Input: part model. Units: mm. Frame: model coordinates. Face numbers are marked on the shaded views. A direction names the side the tool comes from. Round coordinates to 2 decimals unless told otherwise and drop trailing zeros. Order: outer loops, then holes, each group sorted by start corner. A loop starts at its lowest first (then second) coordinate and runs counter-clockwise, first axis right, second up. Notation, with made-up numbers: (-28.5, 73.5) - (5.5, 73.5) arc R21 cw to (5.5, 82.5) - close; hole circle Ø8 at (5, -28.75). An arc over 180 degrees is marked (long way). One line per item, written item: value. Start each with the question number.
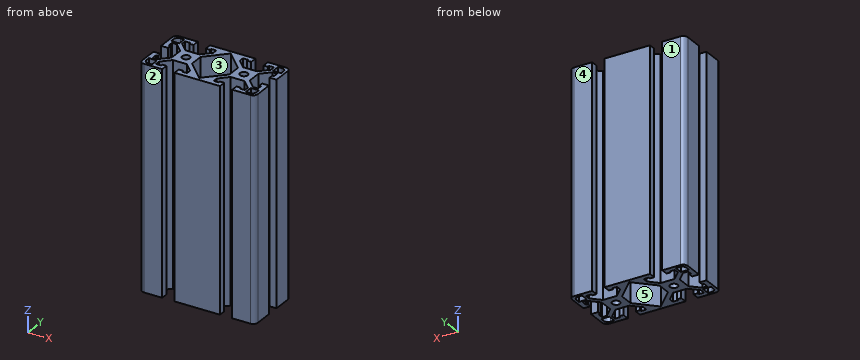
from build123d import *

# Parameters (mm, degrees)
SKETCH1_R           = 2.5527
BOSS_EXTRUDE1_DEPTH = 73.025


with BuildPart() as part:
    # Sketch1 → Boss-Extrude1 (new, symmetric)
    with BuildSketch(Plane.XY):
        with BuildLine():
            Line((-29.337, 12.442261469), (-29.337, 15.6718))
            Line((-29.337, 15.6718), (-25.908, 15.6718))
            Line((-25.908, 15.6718), (-25.908, 14.5034))
            Line((-25.908, 14.5034), (-23.114, 14.5034))
            Line((-23.114, 14.5034), (-23.114, 19.05))
            Line((-23.114, 19.05), (-35.052, 19.05))
            ThreePointArc((-35.052, 19.05), (-37.207261469, 18.157261469), (-38.1, 16.002))
            Line((-38.1, 16.002), (-38.1, 4.064))
            Line((-38.1, 4.064), (-33.5534, 4.064))
            Line((-33.5534, 4.064), (-33.5534, 6.858))
            Line((-33.5534, 6.858), (-34.7218, 6.858))
            Line((-34.7218, 6.858), (-34.7218, 10.287))
            Line((-34.7218, 10.287), (-31.492261469, 10.287))
            Line((-31.492261469, 10.287), (-25.781, 4.575738531))
            Line((-25.781, 4.575738531), (-25.781, -4.575738531))
            Line((-25.781, -4.575738531), (-31.492261469, -10.287))
            Line((-31.492261469, -10.287), (-34.7218, -10.287))
            Line((-34.7218, -10.287), (-34.7218, -6.858))
            Line((-34.7218, -6.858), (-33.5534, -6.858))
            Line((-33.5534, -6.858), (-33.5534, -4.064))
            Line((-33.5534, -4.064), (-38.1, -4.064))
            Line((-38.1, -4.064), (-38.1, -16.002))
            ThreePointArc((-38.1, -16.002), (-37.207261469, -18.157261469), (-35.052, -19.05))
            Line((-35.052, -19.05), (-23.114, -19.05))
            Line((-23.114, -19.05), (-23.114, -14.5034))
            Line((-23.114, -14.5034), (-25.908, -14.5034))
            Line((-25.908, -14.5034), (-25.908, -15.6718))
            Line((-25.908, -15.6718), (-29.337, -15.6718))
            Line((-29.337, -15.6718), (-29.337, -12.442261469))
            Line((-29.337, -12.442261469), (-23.625738531, -6.731))
            Line((-23.625738531, -6.731), (-14.474261469, -6.731))
            Line((-14.474261469, -6.731), (-8.763, -12.442261469))
            Line((-8.763, -12.442261469), (-8.763, -15.6718))
            Line((-8.763, -15.6718), (-12.192, -15.6718))
            Line((-12.192, -15.6718), (-12.192, -14.5034))
            Line((-12.192, -14.5034), (-14.986, -14.5034))
            Line((-14.986, -14.5034), (-14.986, -19.05))
            Line((-14.986, -19.05), (14.986, -19.05))
            Line((14.986, -19.05), (14.986, -14.5034))
            Line((14.986, -14.5034), (12.192, -14.5034))
            Line((12.192, -14.5034), (12.192, -15.6718))
            Line((12.192, -15.6718), (8.763, -15.6718))
            Line((8.763, -15.6718), (8.763, -12.442261469))
            Line((8.763, -12.442261469), (14.474261469, -6.731))
            Line((14.474261469, -6.731), (23.625738531, -6.731))
            Line((23.625738531, -6.731), (29.337, -12.442261469))
            Line((29.337, -12.442261469), (29.337, -15.6718))
            Line((29.337, -15.6718), (25.908, -15.6718))
            Line((25.908, -15.6718), (25.908, -14.5034))
            Line((25.908, -14.5034), (23.114, -14.5034))
            Line((23.114, -14.5034), (23.114, -19.05))
            Line((23.114, -19.05), (35.052, -19.05))
            ThreePointArc((35.052, -19.05), (37.207261469, -18.157261469), (38.1, -16.002))
            Line((38.1, -16.002), (38.1, -4.064))
            Line((38.1, -4.064), (33.5534, -4.064))
            Line((33.5534, -4.064), (33.5534, -6.858))
            Line((33.5534, -6.858), (34.7218, -6.858))
            Line((34.7218, -6.858), (34.7218, -10.287))
            Line((34.7218, -10.287), (31.492261469, -10.287))
            Line((31.492261469, -10.287), (25.781, -4.575738531))
            Line((25.781, -4.575738531), (25.781, 4.575738531))
            Line((25.781, 4.575738531), (31.492261469, 10.287))
            Line((31.492261469, 10.287), (34.7218, 10.287))
            Line((34.7218, 10.287), (34.7218, 6.858))
            Line((34.7218, 6.858), (33.5534, 6.858))
            Line((33.5534, 6.858), (33.5534, 4.064))
            Line((33.5534, 4.064), (38.1, 4.064))
            Line((38.1, 4.064), (38.1, 16.002))
            ThreePointArc((38.1, 16.002), (37.207261469, 18.157261469), (35.052, 19.05))
            Line((35.052, 19.05), (23.114, 19.05))
            Line((23.114, 19.05), (23.114, 14.5034))
            Line((23.114, 14.5034), (25.908, 14.5034))
            Line((25.908, 14.5034), (25.908, 15.6718))
            Line((25.908, 15.6718), (29.337, 15.6718))
            Line((29.337, 15.6718), (29.337, 12.442261469))
            Line((29.337, 12.442261469), (23.625738531, 6.731))
            Line((23.625738531, 6.731), (14.474261469, 6.731))
            Line((14.474261469, 6.731), (8.763, 12.442261469))
            Line((8.763, 12.442261469), (8.763, 15.6718))
            Line((8.763, 15.6718), (12.192, 15.6718))
            Line((12.192, 15.6718), (12.192, 14.5034))
            Line((12.192, 14.5034), (14.986, 14.5034))
            Line((14.986, 14.5034), (14.986, 19.05))
            Line((14.986, 19.05), (-14.986, 19.05))
            Line((-14.986, 19.05), (-14.986, 14.5034))
            Line((-14.986, 14.5034), (-12.192, 14.5034))
            Line((-12.192, 14.5034), (-12.192, 15.6718))
            Line((-12.192, 15.6718), (-8.763, 15.6718))
            Line((-8.763, 15.6718), (-8.763, 12.442261469))
            Line((-8.763, 12.442261469), (-14.474261469, 6.731))
            Line((-14.474261469, 6.731), (-23.625738531, 6.731))
            Line((-23.625738531, 6.731), (-29.337, 12.442261469))
        make_face()
        with Locations((-19.05, 0)):
            Circle(SKETCH1_R, mode=Mode.SUBTRACT)
        with Locations((19.05, 0)):
            Circle(SKETCH1_R, mode=Mode.SUBTRACT)
        Polygon((-12.319, 4.575738531), (-12.319, -4.575738531), (0, -16.894738531), (12.319, -4.575738531), (12.319, 4.575738531), (0, 16.894738531), align=None, mode=Mode.SUBTRACT)
        with BuildLine():
            Line((-30.9372, 11.8872), (-30.9372, 17.272))
            Line((-30.9372, 17.272), (-33.528, 17.272))
            ThreePointArc((-33.528, 17.272), (-35.503656347, 16.453656347), (-36.322, 14.478))
            Line((-36.322, 14.478), (-36.322, 11.8872))
            Line((-36.322, 11.8872), (-30.9372, 11.8872))
        make_face(mode=Mode.SUBTRACT)
        with BuildLine():
            Line((-30.9372, -17.272), (-30.9372, -11.8872))
            Line((-30.9372, -11.8872), (-36.322, -11.8872))
            Line((-36.322, -11.8872), (-36.322, -14.478))
            ThreePointArc((-36.322, -14.478), (-35.503656347, -16.453656347), (-33.528, -17.272))
            Line((-33.528, -17.272), (-30.9372, -17.272))
        make_face(mode=Mode.SUBTRACT)
        with BuildLine():
            Line((36.322, -11.8872), (30.9372, -11.8872))
            Line((30.9372, -11.8872), (30.9372, -17.272))
            Line((30.9372, -17.272), (33.528, -17.272))
            ThreePointArc((33.528, -17.272), (35.503656347, -16.453656347), (36.322, -14.478))
            Line((36.322, -14.478), (36.322, -11.8872))
        make_face(mode=Mode.SUBTRACT)
        with BuildLine():
            Line((30.9372, 17.272), (30.9372, 11.8872))
            Line((30.9372, 11.8872), (36.322, 11.8872))
            Line((36.322, 11.8872), (36.322, 14.478))
            ThreePointArc((36.322, 14.478), (35.503656347, 16.453656347), (33.528, 17.272))
            Line((33.528, 17.272), (30.9372, 17.272))
        make_face(mode=Mode.SUBTRACT)
    extrude(amount=BOSS_EXTRUDE1_DEPTH, both=True)


solid = part.part
Item 1: First-contact query: pin 1 Ø3.5 at (y, z) = (18, -25.5) entering from -X; pin 2 Ø4.5 at (x, z) = (-20.5, 10) entering from -Y; pin 3 Ø2.5 at (y, z) = (-2.5, 8) entering from -X. Flat tips, straight axial feed; report the tip coordinate or a pass-through.
Item 2: Section query B-B on y = 0. Return loops of the section in (x, z) (3 decimals).
Item 3: Section query C-C on z = -32.5. Give the number of separate pieces and of enclosed holes in the cut face, and give its area (3 significant figures).
Item 4: Line query: L1, parallel to Y at x = 33, z = 40; L2, parallel to Y at x = 14.5, z = 4.5; L3, parallel to Y at x = -19, z = 13. Output: solid intervals per line, ascending.
Item 5: Pull-direction query (Y, two-part tool) for the marked faces 1, 2 and 3; classes: released by +Y, released by -Y, zero draft, split by the parting line, or undercut.
Item 6: Section query D-D on x = -4. Return loops of the section in (y, z) (3 decimals), and give its area (3 significant figures).
Item 7: Section query A-A on x = 19.05. Return loops of the section in (y, z) (3 decimals).
Item 8: Reachability of the marked faces 4 and 5 from +Z, -Z, +X, -X, +Y, -Y: full face, straight path, thin tool, end or side. Return the list, or none.
Geometry results:
1. pin 1: stops at x = -38.09
1. pin 2: stops at y = -6.73
1. pin 3: stops at x = -25.78
2. outline: (-25.781, -73.025) - (-21.603, -73.025) - (-21.603, 73.025) - (-25.781, 73.025) - close; (-16.497, -73.025) - (-12.319, -73.025) - (-12.319, 73.025) - (-16.497, 73.025) - close; (12.319, -73.025) - (16.497, -73.025) - (16.497, 73.025) - (12.319, 73.025) - close; (21.603, -73.025) - (25.781, -73.025) - (25.781, 73.025) - (21.603, 73.025) - close
3. separate pieces: 1
3. enclosed holes: 7
3. area: 1,180 mm^2
4. L1: y = -19.05 to -17.27, -11.89 to -10.29, 10.29 to 11.89, 17.27 to 19.05
4. L2: y = -19.05 to -14.5, -6.73 to 6.73, 14.5 to 19.05
4. L3: y = -6.73 to -2.55, 2.55 to 6.73
5. face 1: released by +Y
5. face 2: released by -Y
5. face 3: undercut
6. outline: (-19.05, -73.025) - (-12.895, -73.025) - (-12.895, 73.025) - (-19.05, 73.025) - close; (12.895, -73.025) - (19.05, -73.025) - (19.05, 73.025) - (12.895, 73.025) - close
6. area: 1,800 mm^2
7. outline: (-6.731, -73.025) - (-2.553, -73.025) - (-2.553, 73.025) - (-6.731, 73.025) - close; (2.553, -73.025) - (6.731, -73.025) - (6.731, 73.025) - (2.553, 73.025) - close
8. face 4: +Z, -Z, +X, -X, +Y
8. face 5: +Z, -Z
